from build123d import *

# Parameters (mm, degrees)
BOSS_EXTRUDE1_DEPTH = 3
SKETCH2_R           = 0.25
BOSS_EXTRUDE2_DEPTH = 6


with BuildPart() as part:
    # Sketch1 → Boss-Extrude1 (new body)
    with BuildSketch(Plane(origin=(0, 0, 0), x_dir=(1, 0, 0), z_dir=(0, 1, 0))):
        with BuildLine():
            Line((-2, 3.75), (2, 3.75))
            ThreePointArc((2, 3.75), (2.353553391, 3.603553391), (2.5, 3.25))
            Line((2.5, 3.25), (2.5, -3.25))
            ThreePointArc((2.5, -3.25), (2.353553391, -3.603553391), (2, -3.75))
            Line((2, -3.75), (-2, -3.75))
            ThreePointArc((-2, -3.75), (-2.353553391, -3.603553391), (-2.5, -3.25))
            Line((-2.5, -3.25), (-2.5, 3.25))
            ThreePointArc((-2.5, 3.25), (-2.353553391, 3.603553391), (-2, 3.75))
        make_face()
    extrude(amount=BOSS_EXTRUDE1_DEPTH)

    # Sketch2 → Boss-Extrude2 (add)
    with BuildSketch(Plane(origin=(0, 3, 0), x_dir=(1, 0, 0), z_dir=(0, 1, 0))):
        with Locations((-1.25, 2.875448281)):
            Circle(SKETCH2_R)
        with Locations((1.25, 2.875448281)):
            Circle(SKETCH2_R)
        with Locations((-1.25, -0.124551719)):
            Circle(SKETCH2_R)
        with Locations((1.25, -0.124551719)):
            Circle(SKETCH2_R)
        with Locations((-1.25, -3.124551719)):
            Circle(SKETCH2_R)
        with Locations((1.25, -3.124551719)):
            Circle(SKETCH2_R)
    extrude(amount=BOSS_EXTRUDE2_DEPTH)


solid = part.part
Source: CAD feature listing. Evaluate the final solid. Frame: model axes, mm. A direction names the side the tool comes from. Round coordinates to 2 decimals unless told otherwise and drop trailing zeros. Loops run counter-clockwise (first coordinate to the right, second up) from the corner with the lowest first, then second, coordinate; pieces in that order, holes last. Notation, with made-up numbers: M 41.5,7.25 L 81.5,7.25 A29 ccw 81.5,30.25 Z; hole C -13,-27.5 d4. An arc over 180 degrees is marked long. Return JSON: item names as keys, results as strings. Group by question number.
1. Section query D-D on x = -0.25. Output: boundary loops of the cut face in (y, z), and give its area (3 significant figures).
2. Material intervals for line 1 along Y through (x, z) = (-0.4, -2); line 2 along X through (y, z) = (5.5, 0.25), sorted ascending. Write a range as from..to.
3. Section query B-B on y = 7.25. Output: boundary loops of the cut face in (x, z).
4. Reachability of faces 1 (the face through (0, 1, 3.75)), 2 (the face through (0, 3, 0)) from +Z, -Z, +X, -X, +Y, -Y: full face, straight path, thin tool, end or side. Return the list, or none.
5. Pin query (flat end, axial travel): pin 1 (3 mm diameter, centred on y = 6, z = 2.5, fed in from +X). Return the tip coordinate at first contact, or that it passes through.
6. Section query A-A on x = -1.25. Output: boundary loops of the cut face in (y, z).
7. Section query C-C on z = -1.5. Output: boundary loops of the cut face in (x, y).
Checks:
{
 "1": {"outline": "M 0,-3.75 L 3,-3.75 L 3,3.75 L 0,3.75 Z", "area": "22.5 mm²"},
 "2": {"line 1": "y = 0..3", "line 2": "x = -1.47..-1.03, 1.03..1.47"},
 "3": {"outline": "C -1.25,-2.88 d0.5; C -1.25,0.12 d0.5; C -1.25,3.12 d0.5; C 1.25,-2.88 d0.5; C 1.25,0.12 d0.5; C 1.25,3.12 d0.5"},
 "4": {"face 1": "+Z, +X, -X, +Y, -Y", "face 2": "+Y"},
 "5": {"pin 1": "stops at x = 1.5"},
 "6": {"outline": "M 0,-3.75 L 3,-3.75 L 3,-3.13 L 9,-3.13 L 9,-2.63 L 3,-2.63 L 3,-0.13 L 9,-0.13 L 9,0.37 L 3,0.37 L 3,2.87 L 9,2.87 L 9,3.37 L 3,3.37 L 3,3.75 L 0,3.75 Z"},
 "7": {"outline": "M -2.5,0 L 2.5,0 L 2.5,3 L -2.5,3 Z"}
}
